Autodesk Inventor part; units mm, degrees
ref_plane "YZ Plane" through (0, 0, 0) normal (1, 0, 0) x (0, 1, 0)
ref_plane "XZ Plane" through (0, 0, 0) normal (0, 1, 0) x (-1, 0, 0)
ref_plane "XY Plane" through (0, 0, 0) normal (0, 0, 1) x (1, 0, 0)
sketch "Esquisse1" plane through (0, 0, 0) normal (0, 1, 0) x (-1, 0, 0)
  line L0 (0, 0) -> (15, 0)
  line L1 (15, 0) -> (15, -50)
  line L2 (15, -50) -> (0, -50)
  line L3 (0, -50) -> (0, 0)
  dimension "d0" = 50
  dimension "d1" = 15
extrude "Extrusion1" add sketch "Esquisse1" along normal blind 3
sketch "Esquisse2" plane through (0, 3, 0) normal (0, 1, 0) x (1, 0, 0)
  line L0 (-15, 50) -> (-15, 0)
  line L1 (-15, 11.75) -> (0, 11.75)
  line L2 (0, 11.75) -> (0, 38.25)
  line L3 (0, 38.25) -> (-15, 38.25)
  line L4 (-15, 38.25) -> (-15, 11.75)
  line L5 (-15, 0) -> (0, 0)
  line L6 (0, 50) -> (-15, 50)
  line L7 (-15, 11.75) -> (0, 11.75)
  line L8 (0, 11.75) -> (0, 16.75)
  line L9 (0, 16.75) -> (-15, 16.75)
  line L10 (-15, 16.75) -> (-15, 11.75)
  line L11 (-15, 33.25) -> (0, 33.25)
  line L12 (0, 33.25) -> (0, 38.25)
  line L13 (0, 38.25) -> (-15, 38.25)
  line L14 (-15, 38.25) -> (-15, 33.25)
  dimension "d4" = 15
  dimension "d5" = 11.75
  dimension "d6" = 11.75
  dimension "d7" = 5
  dimension "d8" = 5
extrude "Extrusion2" add sketch "Esquisse2" along normal blind 21 contours L3 L2 L11 L0 | L9 L2 L1 L0
sketch "Esquisse3" plane through (-15, 3, -11.75) normal (0, 0, 1) x (1, 0, 0)
  line L0 (0, 0) -> (15, 0)
  line L1 (0, 0) -> (0, 21)
  point P0 (15, -3)
  point P1 (7.5, 12)
  dimension "d11" = 12
  dimension "d12" = 7.5
hole "Perçage1" at (-7.5, 15, -11.75) direction (0, 0, -1) diameter 8.3 depth 100 tip angle 118
fillet "Congé1" radius 4 1 edges at (0, 24, -14.25)
fillet "Congé2" radius 4 1 edges at (-15, 24, -14.25)
fillet "Congé3" radius 4 1 edges at (-15, 24, -35.75)
fillet "Congé4" radius 4 1 edges at (0, 24, -35.75)
sketch "Esquisse4" plane through (0, 3, 0) normal (0, 1, 0) x (1, 0, 0)
  line L0 (0, 50) -> (0, 0)
  line L1 (-15, 0) -> (0, 0)
  line L2 (0, 0) -> (0, 11.75)
  line L3 (0, 11.75) -> (-15, 11.75)
  line L4 (-15, 11.75) -> (-15, 0)
  line L5 (-15, 0) -> (-15, 50)
  line L6 (-15, 38.25) -> (0, 38.25)
  line L7 (-15, 50) -> (0, 50)
  line L8 (0, 50) -> (0, 38.25)
  line L9 (0, 38.25) -> (-15, 38.25)
  line L10 (-15, 38.25) -> (-15, 50)
  dimension "d24" = 11.75
  dimension "d25" = 15
extrude "Extrusion3" add sketch "Esquisse4" along normal blind 4 contours L0 L6 L5 L7 | L0 L1 L4 L3
fillet "Congé5" radius 2 1 edges at (-7.5, 7, 0)
fillet "Congé6" radius 2 1 edges at (-7.5, 7, -50)
fillet "Congé7" radius 2 3 edges at (0, 7, -43.125) (0, 6.4142, -49.4142) (0, 2.5, -50)
fillet "Congé8" radius 2 3 edges at (0, 7, -6.875) (0, 6.4142, -0.5858) (0, 2.5, 0)
fillet "Congé9" radius 2 3 edges at (-15, 7, -6.875) (-15, 6.4142, -0.5858) (-15, 2.5, 0)
fillet "Congé10" radius 2 3 edges at (-15, 7, -43.125) (-15, 6.4142, -49.4142) (-15, 2.5, -50)
sketch "Esquisse5" plane through (0, 7, 0) normal (0, 1, 0) x (1, 0, 0)
  line L0 (-2, 50) -> (-13, 50)
  line L1 (0, 38.25) -> (0, 48)
  line L2 (0, 2) -> (0, 11.75)
  line L3 (-13, 0) -> (-2, 0)
  point P0 (0, 0)
  point P1 (-7.5, 45)
  point P2 (-7.5, 5)
  dimension "d34" = 5
  dimension "d35" = 7.5
  dimension "d36" = 7.5
  dimension "d37" = 5
hole "Perçage2" at (-7.5, 7, -45) at (-7.5, 7, -5) direction (0, -1, 0) diameter 4.2 depth 100 tip angle 118 countersink diameter 6.5 countersink angle 90
properties part number "support_roue_bascule"
Check sheet for the modelled part. Datum: model origin and axes. Units: mm. A direction names the side the tool comes from. Coordinates: 2 decimals unless noted, no trailing zeros. Loops run counter-clockwise (first coordinate to the right, second up) from the corner with the lowest first, then second, coordinate; pieces in that order, holes last. Notation, with made-up numbers: M 43.25,26.25 L 75.25,26.25 A7 cw 75.25,32.25 Z; hole C 32.5,-21 d8. An arc over 180 degrees is marked long. Answer as a JSON object with one key per item and string values.
1. Access from +Z, -Z, +X, -X, +Y, -Y to the whole of each face (thin tool, end or side, straight path). Record for faces 1 (the flat face through (-8, 7, -9)), 2 (the cylindrical face through (-0.57, 6.4, -6.81)), 3 (the cylindrical face through (-0.57, 6.4, -43.06)), 4 (the flat face through (-5.7, 11, -16.75)).
Outcome:
{"face 1": "+Z, +X, -X, +Y", "face 2": "+Z, +X, +Y", "face 3": "-Z, +X, +Y", "face 4": "+X, -X, +Y"}
2. Release check for a two-part mould opening along Z. For faces 5 (the flat face through (-5.9, 11, -33.25)), 6 (the cylindrical face through (-1.203, 22.859, -14.285)), 7 (the flat face through (-11, 12, -11.75)) record: pulls with the +Z half, pulls with the -Z half, needs draft (parallel to the pull), parting line crosses it, or undercut.
Outcome:
{"face 5": "undercut", "face 6": "needs draft", "face 7": "pulls with the +Z half"}
3. Sectioned sample at D-D on z = -37. Record the cut outline in (x, y).
Outcome:
{"outline": "M -15,0 L 0,0 L 0,20 A4 ccw -4,24 L -11,24 A4 ccw -15,20 Z; hole C -7.5,15 d8.3"}
4. Scan lines: L1, parallel to Z at x = -7.5, y = 2.3; L2, parallel to Z at x = -8.25, y = 20.5; L3, parallel to Z at x = -7.5, y = 4.7. Record each from-to range of solid material in increasing order. Write a range as from..to.
Outcome:
{"L1": "-50..-47.1, -42.9..-7.1, -2.9..0", "L2": "-38.25..-33.25, -16.75..-11.75", "L3": "-50..-47.1, -42.9..-33.25, -16.75..-7.1, -2.9..0"}
5. Sectioned sample at A-A on y = 15. Record the cut outline in (x, z).
Outcome:
{"outline": "M -15,-38.25 L -11.65,-38.25 L -11.65,-33.25 L -15,-33.25 Z; M -15,-16.75 L -11.65,-16.75 L -11.65,-11.75 L -15,-11.75 Z; M -3.35,-38.25 L 0,-38.25 L 0,-33.25 L -3.35,-33.25 Z; M -3.35,-16.75 L 0,-16.75 L 0,-11.75 L -3.35,-11.75 Z"}
6. Depth check by flat-ended pin: P1, Ø5, axis at x = -6, z = -5, coming from the +Y side; P2, Ø1.5, axis at x = -2.5, z = -14, coming from the +Y side; P3, Ø1, axis at x = -3, z = -28.5, coming from the +Y side. Enter the tip coordinate at first touch or a pass-through.
Outcome:
{"P1": "y = 7", "P2": "y = 23.93", "P3": "y = 3"}
7. Sectioned sample at B-B on z = -45. Record the cut outline in (x, y), and give its area (3 significant figures).
Outcome:
{"outline": "M -15,0 L -9.6,0 L -9.6,5.85 L -10.75,7 L -13,7 A2 ccw -15,5 Z; M -5.4,0 L 0,0 L 0,5 A2 ccw -2,7 L -4.25,7 L -5.4,5.85 Z", "area": "72.6 mm²"}
8. Sectioned sample at C-C on x = -7.5. Count the separate pieces of the cut face and the enclosed holes in it, and give its area (3 significant figures).
Outcome:
{"separate pieces": "5", "enclosed holes": "0", "area": "308 mm²"}
